from build123d import *

# Parameters (mm, degrees)
F0_W     = 355.6
F0_H     = 184.15
F0_W_2   = 203.2
F0_H_2   = 101.6
F1_DEPTH = 19.05
F2_SIZE2 = 19.04999
F2_SIZE  = 19.04999


# Not quite as in the source:
# - a fillet or chamfer is up to 0.001 mm smaller than in the source, because OpenCascade refuses the exact size


with BuildPart() as f1:
    # F0 (on Top) → F1 (new body)
    with BuildSketch(Plane.XY):
        Rectangle(F0_W, F0_H)
        Rectangle(F0_W_2, F0_H_2, mode=Mode.SUBTRACT)
    extrude(amount=F1_DEPTH)

    # F2 (size 19.05 and 19.05 in the source; OpenCascade refuses exactly that, so slightly less here)
    f2_edges = [f1.edges().sort_by_distance(p)[0] for p in [
        (-101.6, 0, 19.05),
        (0, 50.8, 19.05),
        (101.6, 0, 19.05),
        (0, -50.8, 19.05),
    ]]
    chamfer(f2_edges, length=F2_SIZE, length2=F2_SIZE2)


solid = f1.part
Can you work these out from the model? Positions are in its coordinate system, mm. A direction names the side the tool comes from. Round coordinates to 2 decimals unless told otherwise and drop trailing zeros. Loops run counter-clockwise (first coordinate to the right, second up) from the corner with the lowest first, then second, coordinate; pieces in that order, holes last. Notation, with made-up numbers: (69.25, 72) - (105.25, 72) arc R23 cw to (105.25, 80) - close; hole circle Ø3 at (56, -27.75). An arc over 180 degrees is marked (long way). Answer in a Markdown table with one row per item. Add a question column.
Q1. I want a section at C-C on z = 12. List the corners of the cut face in (x, y) for me (3 decimals), and give its area (3 significant figures).
Q2. We'd pull the mould along X, two halves only. Please class faces 3 (the flat face through (-177.8, -1, 9)), 4 (the flat face through (-1.7, -60.5, 9.7)), 5 (the flat face through (177.8, -1, 9)), 6 (the flat face through (-42, -81, 19.05)): pulls with the +X half, pulls with the -X half, needs draft (parallel to the pull), parting line crosses it, or undercut.
Q3. I want a section at D-D on x = -111.5. List the corners of the cut face in (y, z) for me (3 decimals).
Q4. I need wall thicknesses on L1, parallel to Y at x = 54.5, z = 3 (3 decimals); L2, parallel to X at y = 30, z = 10.5; L3, parallel to Y at x = 69, z = 11.5 (3 decimals). Which ranges of each line are inside material? Lowest first, please.
Q5. Which directions (+Z, -Z, +X, -X, +Y, -Y) give clear straight access to the entire face, cutting with the end or side of a thin tool? Please do faces 1 (the flat face through (-111.3, -1, 9.7)), 2 (the flat face through (-2, 63, 0)).
A:
| question | item | result |
|---|---|---|
| 1 | outline | (-177.8, -92.075) - (177.8, -92.075) - (177.8, 92.075) - (-177.8, 92.075) - close; hole (-113.6, -62.8) - (113.6, -62.8) - (113.6, 62.8) - (-113.6, 62.8) - close |
| 1 | area | 36,900 mm^2 |
| 2 | face 3 | pulls with the -X half |
| 2 | face 4 | undercut |
| 2 | face 5 | pulls with the +X half |
| 2 | face 6 | needs draft |
| 3 | outline | (-92.075, 0) - (92.075, 0) - (92.075, 19.05) - (69.85, 19.05) - (60.7, 9.9) - (-60.7, 9.9) - (-69.85, 19.05) - (-92.075, 19.05) - close |
| 4 | L1 | -92.075 to -53.8, 53.8 to 92.075 |
| 4 | L2 | -177.8 to -112.1, 112.1 to 177.8 |
| 4 | L3 | -92.075 to -62.3, 62.3 to 92.075 |
| 5 | face 1 | +Z |
| 5 | face 2 | -Z, +X, -X, +Y, -Y |
